Here's the drawing with two shaded views (mm, measured from the low corner). I have some questions. A direction names the side the tool comes from. Coordinates: 2 decimals unless noted, no trailing zeros. Write each loop counter-clockwise with the first axis right and the second up, starting at its lowest first coordinate (ties: lowest second). Pieces come first, ordered by that corner, then holes. Notation, with made-up numbers: (14, 77) -> (50, 77) arc R18 ccw to (50, 110) -> close; hole circle Ø4 at (17.5, -6.75). An arc over 180 degrees is marked (long way). Put each result on its own line as item: value. Start each with the question number.
Item 1: I want a section at B-B, the plane z = 61.5. List the corners of the cut face in (x, y) for me.
Item 2: For pin 1 (3 mm diameter, centred on x = 37, z = 76.5, fed in from -Y); pin 2 (12 mm diameter, centred on x = 10.5, z = 19, fed in from +Y); pin 3 (10 mm diameter, centred on y = 19.5, z = 36.5, fed in from +X); pin 4 (12 mm diameter, centred on y = 17, z = 33, fed in from -X), each with a flat end and sliding along its axis, tell me the tip position at first contact or that it passes through.
Item 3: If we mould it in two halves opening along X, with no side actions, what happens to the marked faces 1 and 2? For each: released by +X, released by -X, zero draft, split by the parting line, or undercut.
Item 4: I need wall thicknesses on line 1 (Z direction, x = 8, y = 13.25); line 2 (Y direction, x = 94.5, z = 20.5); line 3 (X direction, y = 12.5, z = 89) (1 decimal). Which ranges of each line are inside material? Lowest first, please. Write a range as [from, to].
Item 5: I want a section at A-A, the plane y = 13.75. State how many separate pieces and enclosed holes the cut face has.
Item 6: On a 3-axis mill with a long thin cutter (end or side, diameter ignored), from which of +Z, -Z, +X, -X, +Y, -Y can I reach the whole of each face in a straight line? I mean the marked faces 3 and 4. Say none if no direction works.
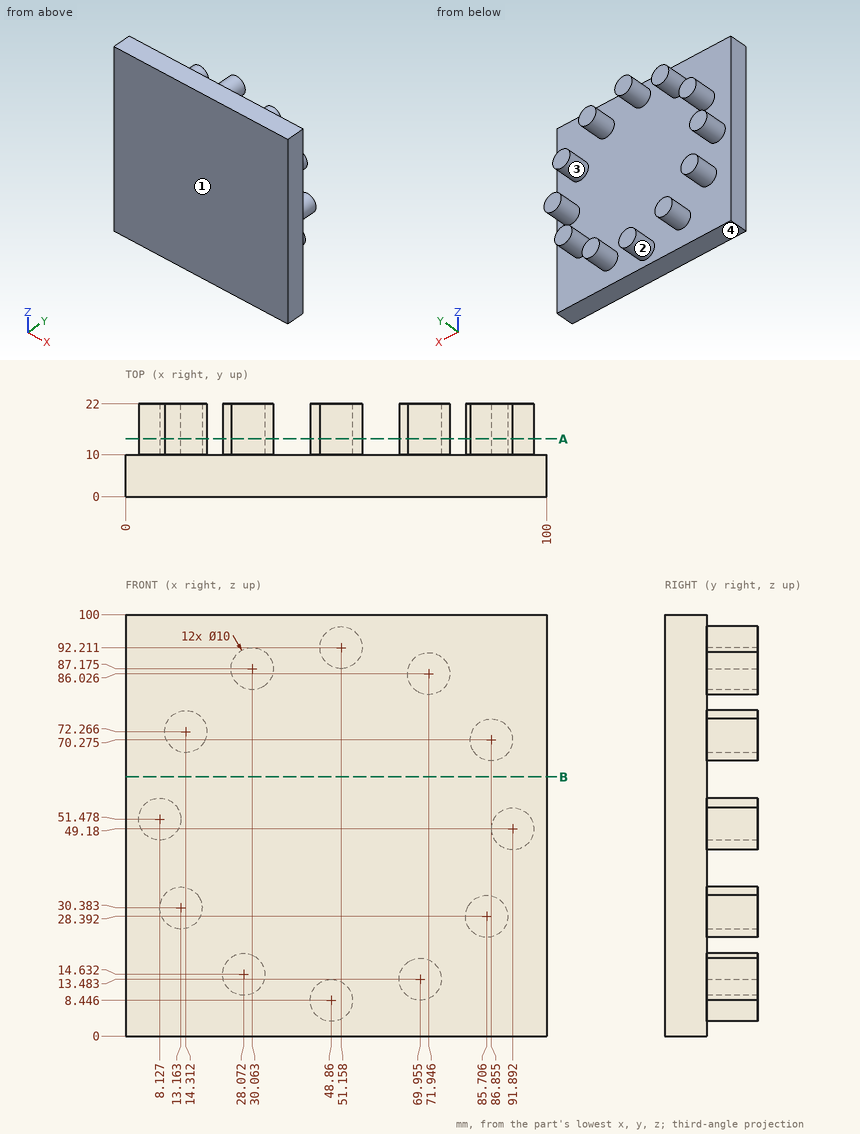
Calculated:
1. outline: (0, 0) -> (100, 0) -> (100, 10) -> (0, 10) -> close
2. pin 1: stops at y = 0
2. pin 2: stops at y = 10
2. pin 3: stops at x = 89.62
2. pin 4: stops at x = 8.16
3. face 1: zero draft
3. face 2: undercut
4. line 1: z = [46.48, 56.48]
4. line 2: y = [0, 10]
4. line 3: x = [25.4, 34.7], [47.3, 55], [67.9, 76]
5. separate pieces: 12
5. enclosed holes: 0
6. face 3: +Y
6. face 4: -Z, +X, -X, +Y, -Y
